```python
from build123d import *

# Parameters (mm, degrees)
SKETCH1_W           = 11
SKETCH1_H           = 18
SKETCH1_W_2         = 5
SKETCH1_H_2         = 11
BOSS_EXTRUDE1_DEPTH = 4
BOSS_EXTRUDE2_DEPTH = 5
SKETCH3_R           = 1.248430758
CUT_EXTRUDE1_DEPTH  = 5
FILLET1_R           = 1
FILLET3_R           = 2
FILLET4_R           = 9
CUT_EXTRUDE2_DEPTH  = 10
CHAMFER2_SIZE       = 1


with BuildPart() as part:
    # Sketch1 → Boss-Extrude1 (new body)
    with BuildSketch(Plane(origin=(0, 0, 0), x_dir=(1, 0, 0), z_dir=(0, 1, 0))):
        with Locations((-2.740875912, 16.357664234)):
            Rectangle(SKETCH1_W, SKETCH1_H)
        with Locations((-5.740875912, 30.857664234)):
            Rectangle(SKETCH1_W_2, SKETCH1_H_2)
    boss_extrude1 = extrude(amount=BOSS_EXTRUDE1_DEPTH)

    # Sketch2 → Boss-Extrude2 (add)
    with BuildSketch(Plane(origin=(-3.240875912, 0, 0), x_dir=(0, 0, -1), z_dir=(1, 0, 0))):
        with BuildLine():
            Line((34.537911903, 0), (25.357664234, 0))
            Line((25.357664234, 0), (25.357664234, -12.192130501))
            Line((25.357664234, -12.192130501), (34.537911903, -12.192130501))
            Line((34.537911903, -12.192130501), (34.537911903, -7.165523267))
            ThreePointArc((34.537911903, -7.165523267), (33.357664234, -5.7), (34.537911903, -4.234476733))
            Line((34.537911903, -4.234476733), (34.537911903, 0))
        make_face()
        with BuildLine():
            Line((36.357664234, 0), (34.537911903, 0))
            Line((34.537911903, 0), (34.537911903, -4.234476733))
            ThreePointArc((34.537911903, -4.234476733), (35.798507341, -4.531747353), (36.357664234, -5.7))
            ThreePointArc((36.357664234, -5.7), (35.798507341, -6.868252647), (34.537911903, -7.165523267))
            Line((34.537911903, -7.165523267), (34.537911903, -12.192130501))
            ThreePointArc((34.537911903, -12.192130501), (41.293121094, -6.613725887), (36.357664234, 0.62455532))
            Line((36.357664234, 0.62455532), (36.357664234, 0))
        make_face()
    boss_extrude2 = extrude(amount=-BOSS_EXTRUDE2_DEPTH)

    # Mirror1: Boss-Extrude1, Boss-Extrude2 across plane
    add(boss_extrude1.mirror(Plane(origin=(-8.240875912, 4, 0), x_dir=(0, 0, 1), z_dir=(1, 0, 0))))
    add(boss_extrude2.mirror(Plane(origin=(-8.240875912, 4, 0), x_dir=(0, 0, 1), z_dir=(1, 0, 0))))

    # Sketch3 → Cut-Extrude1 (cut)
    with BuildSketch(Plane(origin=(0, 4, 0), x_dir=(1, 0, 0), z_dir=(0, 1, 0))):
        with Locations(Location((-8.240875912, 15.357664234, 0), (0, 0, 270))):
            Circle(SKETCH3_R)
    extrude(amount=-CUT_EXTRUDE1_DEPTH, mode=Mode.SUBTRACT)

    # Fillet1
    fillet1_edges = [part.edges().sort_by_distance(p)[0] for p in [
        (-0.240875912, 4, -25.357664234),
        (-3.240875912, -4.234476733, -35.177416564),
        (-8.240875912, 4, -7.357664234),
        (-19.240875912, 4, -16.357664234),
        (-16.240875912, 4, -25.357664234),
        (2.759124088, 4, -16.357664234),
        (-13.240875912, -4.234476733, -35.177416564),
    ]]
    fillet(fillet1_edges, radius=FILLET1_R)

    # Fillet3
    fillet3_edges = [part.edges().sort_by_distance(p)[0] for p in [
        (-8.240875912, 0, -25.357664234),
    ]]
    fillet(fillet3_edges, radius=FILLET3_R)

    # Fillet4
    fillet4_edges = [part.edges().sort_by_distance(p)[0] for p in [
        (-8.240875912, -12.192130501, -25.357664234),
    ]]
    fillet(fillet4_edges, radius=FILLET4_R)

    # Sketch4 → Cut-Extrude2 (cut)
    with BuildSketch(Plane.ZY.offset(13.240875912)):
        Polygon((-36.357664234, 0.62455532), (-24.357664234, 4), (-36.357664234, 4), align=None)
    extrude(amount=-CUT_EXTRUDE2_DEPTH, mode=Mode.SUBTRACT)

    # Chamfer2
    chamfer2_edges = [part.edges().sort_by_distance(p)[0] for p in [
        (-8.240875912, 4, -16.606094992),
    ]]
    chamfer(chamfer2_edges, length=CHAMFER2_SIZE)


solid = part.part
```
Geometry: final body of the model. Coordinates: model frame, mm. A direction names the side the tool comes from. Coordinates: 2 decimals unless noted, no trailing zeros. Order: outer loops, then holes, each group sorted by start corner. A loop starts at its lowest first (then second) coordinate and runs counter-clockwise, first axis right, second up.
Item 1: Access query for faces 5 (the face through (-0.2, 3.7, -25.07)), 6 (the face through (-16, 1, -25.358)), 7 (the face through (-16.28, 3.7, -25.07)). Directions: +Z, -Z, +X, -X, +Y, -Y. A direction counts if a zero-diameter tool reaches every point of the face in a straight line with its end or side. Return the directions, or none.
Answer:
face 5: -Z, +X, +Y
face 6: -Z, -X, +Y, -Y
face 7: -Z, -X, +Y
Item 2: Material intervals for line 1 along Y through (x, z) = (-11.25, -23); line 2 along X through (y, z) = (0.25, -31.5); line 3 along Y through (x, z) = (-7.75, -34), sorted ascending.
Answer:
line 1: y = 0 to 4
line 2: x = -13.24 to -3.24
line 3: y = -12.19 to -6.93, -4.47 to 1.29
Item 3: Section query A-A (x = -11.75). Output: boundary loops of the cut face in (y, z).
Answer:
outline: (-12.19, -34.54) arc R6.5 ccw to (0.62, -36.36) - (4, -24.36) - (4, -8.36) arc R1 ccw to (3, -7.36) - (0, -7.36) - (0, -23.36) arc R2 cw to (-2, -25.36) - (-3.19, -25.36) arc R9 ccw to (-12.19, -34.36) - close; hole circle Ø3 at (-5.7, -34.86)
Item 4: Draft query along X for faces 1 (the face through (-8.186, 1.521, -16.605)), 2 (the face through (-18.956, 3.699, -16.484)), 3 (the face through (-8.171, -9.486, -27.924)), 4 (the face through (2.474, 3.699, -16.484)). Return one class per face: released by +X, released by -X, zero draft, split by the parting line, or undercut.
Answer:
face 1: undercut
face 2: released by -X
face 3: zero draft
face 4: released by +X
Item 5: Section query B-B (y = 2.5). Output: boundary loops of the cut face in (x, z), then the cut area to 3 significant figures.
Answer:
outline: (-19.24, -25.36) - (-13.24, -25.36) - (-13.24, -29.69) - (-3.24, -29.69) - (-3.24, -25.36) - (2.76, -25.36) - (2.76, -7.36) - (-19.24, -7.36) - close; hole circle Ø2.5 at (-8.24, -15.36)
area: 434 mm2
Item 6: Contact query for flat-ended pins moving along their axis: P1, Ø3, axis at x = -10.5, y = -5, coming from the -Z side; P2, Ø2, axis at x = 0.5, y = -2.5, coming from the +Z side; P3, Ø1, axis at x = -10.5, y = -3, coming from the +Z side; P4, Ø1, axis at y = -9, z = -37.5, coming from the -X side. Output: stop coordinate, or through.
Answer:
P1: stops at z = -41.36
P2: passes through
P3: stops at z = -25.36
P4: stops at x = -13.24
Item 7: Section query C-C (z = -24). Output: boundary loops of the cut face in (x, y).
Answer:
outline: (-19.24, 0) - (-13.24, 0) - (-13.24, -0.11) - (-3.24, -0.11) - (-3.24, 0) - (2.76, 0) - (2.76, 3) arc R1 ccw to (1.76, 4) - (-18.24, 4) arc R1 ccw to (-19.24, 3) - close
Item 8: Section query D-D (x = 0.5). Output: boundary loops of the cut face in (y, z), then the cut area to 3 significant figures.
Answer:
outline: (0, -25.36) - (3, -25.36) arc R1 ccw to (4, -24.36) - (4, -8.36) arc R1 ccw to (3, -7.36) - (0, -7.36) - close
area: 71.6 mm2
